```python
from build123d import *
from build123d.topology import SkipClean

# Parameters (mm, degrees)
BOSS_EXTRUDE1_DEPTH   = 14
SKETCH2_R             = 6
BOSS_EXTRUDE2_DEPTH   = 12
BOSS_EXTRUDE3_START   = 15
SKETCH3_R             = 6
BOSS_EXTRUDE3_DEPTH   = 15
CUT_EXTRUDE1_DEPTH    = 2.2
BOSS_EXTRUDE4_START   = 14
BOSS_EXTRUDE4_DEPTH   = 14
CUT_EXTRUDE2_DEPTH    = 10
SKETCH24_R            = 3
CUT_EXTRUDE3_DEPTH    = 2.5
M4_TAPPED_HOLE1_D     = 3.3
M4_TAPPED_HOLE1_DEPTH = 10
M4_TAPPED_HOLE1_TIP   = 0.991420021


with BuildPart() as part:
    # Sketch1 → Boss-Extrude1 (new body)
    with BuildSketch(Plane(origin=(0, 0, 0), x_dir=(1, 0, 0), z_dir=(0, 1, 0))):
        with BuildLine():
            ThreePointArc((5.656854249, 2), (-6, 0), (5.656854249, -2))
            ThreePointArc((5.656854249, -2), (6, 0), (5.656854249, 2))
        make_face()
    extrude(amount=BOSS_EXTRUDE1_DEPTH)

    # Sketch2 → Boss-Extrude2 (add)
    with BuildSketch(Plane(origin=(0, 14, 0), x_dir=(1, 0, 0), z_dir=(0, 1, 0))):
        with Locations(Location((0, 0, 0), (0, 0, 270))):
            Circle(SKETCH2_R)
    extrude(amount=BOSS_EXTRUDE2_DEPTH)

    # Sketch3 → Boss-Extrude3 (add)
    with BuildSketch(Plane.XZ.offset(BOSS_EXTRUDE3_START)):
        with Locations(Location((0, 0, 0), (0, 0, 270))):
            Circle(SKETCH3_R)
    extrude(amount=-BOSS_EXTRUDE3_DEPTH)

    # Groove Sketch → Retaining Ring Groove (revolve, cut)
    with BuildSketch(Plane(origin=(1.604252923, 12.182890291, 0.373259529), x_dir=(-0.9343262431877186, 0.2824476966643587, -0.2173885230174828), z_dir=(-0.2266157025474993, 0, 0.9739842521103221)), mode=Mode.PRIVATE) as retaining_ring_groove_sk:
        with BuildLine():
            Line((10.620148315, -10.234181518), (12.083054432, -9.80344878))
            Line((12.083054432, -9.80344878), (11.800606735, -8.84416608))
            Line((11.800606735, -8.84416608), (10.337700618, -9.274898818))
            ThreePointArc((10.337700618, -9.274898818), (10.21858296, -9.371036434), (10.202333617, -9.523244897))
            Line((10.202333617, -9.523244897), (10.371802235, -10.098814517))
            ThreePointArc((10.371802235, -10.098814517), (10.467939851, -10.217932175), (10.620148315, -10.234181518))
        make_face()
    revolve(retaining_ring_groove_sk.sketch.rotate(Axis((0, 60.224615576, 0), (0, -1, 0)), 76.902094509), axis=Axis((0, 60.224615576, 0), (0, -1, 0)), mode=Mode.SUBTRACT)

    # Sketch21 → Cut-Extrude1 (cut)
    with SkipClean():  # the faces are left unmerged after this step: merging them gives an invalid solid
        with BuildSketch(Plane(origin=(6, 0, 0), x_dir=(0, 0, -1), z_dir=(1, 0, 0))):
            with BuildLine():
                Line((-1, 14), (1, 14))
                ThreePointArc((1, 14), (1.707106781, 13.707106781), (2, 13))
                Line((2, 13), (2, 1))
                ThreePointArc((2, 1), (1.707106781, 0.292893219), (1, 0))
                Line((1, 0), (-1, 0))
                ThreePointArc((-1, 0), (-1.707106781, 0.292893219), (-2, 1))
                Line((-2, 1), (-2, 13))
                ThreePointArc((-2, 13), (-1.707106781, 13.707106781), (-1, 14))
            make_face()
        extrude(amount=-CUT_EXTRUDE1_DEPTH, mode=Mode.SUBTRACT)

    # Sketch22 → Boss-Extrude4 (add)
    with SkipClean():  # the faces are left unmerged after this step: merging them gives an invalid solid
        with BuildSketch(Plane.XZ.offset(15).offset(BOSS_EXTRUDE4_START)):
            with BuildLine():
                ThreePointArc((2.397915762, -5.5), (0, 6), (-2.397915762, -5.5))
                ThreePointArc((-2.397915762, -5.5), (0, -6), (2.397915762, -5.5))
            make_face()
        extrude(amount=-BOSS_EXTRUDE4_DEPTH)

    # Sketch23 → Cut-Extrude2 (cut)
    with SkipClean():  # the faces are left unmerged after this step: merging them gives an invalid solid
        with BuildSketch(Plane.XZ.offset(29)):
            with BuildLine():
                Line((-2.397915762, 5.5), (2.397915762, 5.5))
                ThreePointArc((2.397915762, 5.5), (0, 6), (-2.397915762, 5.5))
            make_face()
        extrude(amount=-CUT_EXTRUDE2_DEPTH, mode=Mode.SUBTRACT)

    # Sketch24 → Cut-Extrude3 (cut)
    with SkipClean():  # the faces are left unmerged after this step: merging them gives an invalid solid
        with BuildSketch(Plane(origin=(0, 26, 0), x_dir=(1, 0, 0), z_dir=(0, 1, 0))):
            with Locations(Location((0, 0, 0), (0, 0, 270))):
                Circle(SKETCH24_R)
        extrude(amount=-CUT_EXTRUDE3_DEPTH, mode=Mode.SUBTRACT)

    # M4 Tapped Hole1
    with Locations(Plane(origin=(0, -29, 0), x_dir=(-1, 0, 0), z_dir=(0, -1, 0))):
        with Locations((0, 0)):
            Hole(M4_TAPPED_HOLE1_D / 2, depth=M4_TAPPED_HOLE1_DEPTH)
            with Locations((0, 0, -(M4_TAPPED_HOLE1_DEPTH + M4_TAPPED_HOLE1_TIP / 2))):  # 118° drill point
                Cone(0, M4_TAPPED_HOLE1_D / 2, M4_TAPPED_HOLE1_TIP, mode=Mode.SUBTRACT)


solid = part.part
```
Work out the finished part from the listing and answer in its coordinate system (mm). A direction names the side the tool comes from. Round coordinates to 2 decimals unless told otherwise and drop trailing zeros. Order: outer loops, then holes, each group sorted by start corner. A loop starts at its lowest first (then second) coordinate and runs counter-clockwise, first axis right, second up.
Q1. A cutting plane is placed at B-B, the plane y = 2. Determine the outline of the cut face in (x, z).
Solution:
outline: (3.8, -2) - (3.8, 2) - (5.66, 2) arc R6 ccw (long way) to (5.66, -2) - close
Q2. The mould has two halves that part along Y. Classify faces 6 (the flat face through (0, 23.5, 0)), 7 (the flat face through (5, 7, -2)), 8 (the cylindrical face through (-1.216, -23.93, -1.115)): pulls with the +Y half, pulls with the -Y half, needs draft (parallel to the pull), parting line crosses it, or undercut.
Solution:
face 6: pulls with the +Y half
face 7: undercut
face 8: needs draft
Q3. A tool of negligible diameter and unlimited length cuts with its end or side. For faces 1 (the flat face through (5, 14, 0)), 2 (the cylindrical face through (0.9, 24.77, 2.86)), 3 (the cylindrical face through (1.802, 25.493, 5.723)), 4 (the cylindrical face through (0.24, 24.504, 5.445)), 5 (the flat face through (0, -24, 5.5)), from which of +Z, -Z, +X, -X, +Y, -Y can it reach the whole face along a straight path? Write none if from no direction.
Solution:
face 1: +X
face 2: +Y
face 3: +Y, -Y
face 4: none
face 5: +Z, +X, -X, -Y
Q4. A cutting plane is placed at A-A, the plane y = -22. Determine the outline of the cut face in (x, z), then the cut area to 3 significant figures.
Solution:
outline: (-2.4, 5.5) arc R6 ccw (long way) to (2.4, 5.5) - close; hole circle Ø3.3 at (0, 0)
area: 103 mm2
Q5. Given pin 1 Ø1.8 at (x, z) = (-1, 0) entering from +Y; pin 2 Ø2.5 at (x, z) = (0, 0) entering from -Y; pin 3 Ø2 at (y, z) = (5.5, 0) entering from +X, each flat-ended and moving along its own axis, determine where each tip first touches the part or whether it passes through.
Solution:
pin 1: stops at y = 23.5
pin 2: stops at y = -18.76
pin 3: stops at x = 3.8
Q6. Find the intervals of material crossed by line 1 along Z through (x, y) = (0, -22.25); line 2 along Y through (x, z) = (-5, -3); line 3 along Z through (x, y) = (2.5, 14), in increasing order.
Solution:
line 1: z = -6 to -1.65, 1.65 to 5.5
line 2: y = -29 to 24, 25 to 26
line 3: z = -5.45 to 5.45
